```python
from build123d import *

# Parameters (mm, degrees)
SKETCH1_R           = 12
BOSS_EXTRUDE1_DEPTH = 10
SKETCH2_R           = 12
BOSS_EXTRUDE2_DEPTH = 10
SKETCH3_R           = 12
BOSS_EXTRUDE3_DEPTH = 10
CUT_EXTRUDE1_DEPTH  = 6


with BuildPart() as part:
    # Sketch1 → Boss-Extrude1 (new body)
    with BuildSketch(Plane(origin=(0, 0, 0), x_dir=(1, 0, 0), z_dir=(0, 1, 0))):
        with Locations(Location((0, 0, 0), (0, 0, 270))):
            Circle(SKETCH1_R)
    extrude(amount=BOSS_EXTRUDE1_DEPTH)

    # Sketch2 → Boss-Extrude2 (add)
    with BuildSketch(Plane(origin=(0, 10, 0), x_dir=(1, 0, 0), z_dir=(0, 1, 0))):
        with Locations(Location((6, 0, 0), (0, 0, 104.477512186))):
            Circle(SKETCH2_R)
    extrude(amount=BOSS_EXTRUDE2_DEPTH)

    # Sketch3 → Boss-Extrude3 (add)
    with BuildSketch(Plane(origin=(0, 20, 0), x_dir=(1, 0, 0), z_dir=(0, 1, 0))):
        with Locations(Location((-6, 0, 0), (0, 0, 60))):
            Circle(SKETCH3_R)
    extrude(amount=BOSS_EXTRUDE3_DEPTH)

    # Sketch4 → Cut-Extrude1 (cut)
    with BuildSketch(Plane.XZ):
        with BuildLine():
            Line((-2.180114967, -2.060849032), (-2.180114967, 2.060849032))
            ThreePointArc((-2.180114967, 2.060849032), (3, 0), (-2.180114967, -2.060849032))
        make_face()
    extrude(amount=-CUT_EXTRUDE1_DEPTH, mode=Mode.SUBTRACT)


solid = part.part
```
The model under review builds one solid part; all positions refer to its coordinate system, in mm. A direction names the side the tool comes from. Give positions to 0.01 mm unless a question says otherwise; leave off trailing zeros. Write each loop counter-clockwise with the first axis right and the second up, starting at its lowest first coordinate (ties: lowest second). Pieces come first, ordered by that corner, then holes. Notation, with made-up numbers: (47, 84) - (72, 84) arc R7 ccw to (72, 90) - close; hole circle Ø6 at (-23, -27.5). An arc over 180 degrees is marked (long way). Answer in a Markdown table with one row per item. Add a question column.
1. We need section A-A on z = 0. Write out the cut boundary in (x, y), then the cut area to 3 significant figures.
2. We need section D-D on z = -8.5. Write out the cut boundary in (x, y).
3. Wall thickness on line 1 along Y through (x, z) = (-3.5, -7.75); line 2 along X through (y, z) = (3.7, 0); line 3 along Y through (x, z) = (4.5, 6): over which ranges is each line inside the solid? List them lowest first. Write a range as [from, to].
4. Tool access review of faces 1 (the cylindrical face through (3.604, 4.93, 11.446)), 2 (the flat face through (13, 10, 0)), 3 (the cylindrical face through (15.451, 14.93, 7.395)), 4 (the flat face through (-2.5, 0, -0.2)), 5 (the flat face through (-8, 10, 0)): name each direction out of +Z, -Z, +X, -X, +Y, -Y from which nothing blocks a thin tool from reaching the whole face with its end or side.
5. We need section C-C on y = 6.5. Write out the cut boundary in (x, z).
6. Draft analysis for pull direction Z (two halves, no side actions). For faces 6 (the cylindrical face through (3, 3, 0)), 7 (the cylindrical face through (2.844, 24.93, 8.11)), 8 (the flat face through (0, 6, 0)), 9 (the flat face through (-6, 30, 0)), state which applies: +Z half, -Z half, draft (parallel to the pull), parting line (faces both ways), or undercut.
7. Insertion check: P1, Ø4, axis at x = 5, y = 6.5, coming from the +Z side; P2, Ø1.6, axis at x = 0, z = 0, coming from the -Y side; P3, Ø5, axis at x = 3, y = 6.5, coming from the -Z side. Each pin has a flat end and moves straight along its axis. Give the tip position at first contact, or say it passes through.
8. We need section B-B on x = 7. Write out the cut boundary in (y, z).
Ans:
| question | item | result |
|---|---|---|
| 1 | outline | (-18, 20) - (-6, 20) - (-6, 10) - (-12, 10) - (-12, 0) - (-2.18, 0) - (-2.18, 6) - (3, 6) - (3, 0) - (12, 0) - (12, 10) - (18, 10) - (18, 20) - (6, 20) - (6, 30) - (-18, 30) - close |
| 1 | area | 689 mm^2 |
| 2 | outline | (-14.47, 20) - (-2.47, 20) - (-2.47, 10) - (-8.47, 10) - (-8.47, 0) - (8.47, 0) - (8.47, 10) - (14.47, 10) - (14.47, 20) - (2.47, 20) - (2.47, 30) - (-14.47, 30) - close |
| 3 | line 1 | y = [0, 10], [20, 30] |
| 3 | line 2 | x = [-12, -2.18], [3, 12] |
| 3 | line 3 | y = [0, 20] |
| 4 | face 1 | -Y |
| 4 | face 2 | +X, -Y |
| 4 | face 3 | none |
| 4 | face 4 | +Z, -Z, +X, -X, -Y |
| 4 | face 5 | -X |
| 5 | outline | circle Ø24 at (0, 0) |
| 6 | face 6 | undercut |
| 6 | face 7 | parting line |
| 6 | face 8 | undercut |
| 6 | face 9 | draft |
| 7 | P1 | stops at z = 11.62 |
| 7 | P2 | stops at y = 6 |
| 7 | P3 | stops at z = -11.99 |
| 8 | outline | (0, -9.75) - (10, -9.75) - (10, -11.96) - (20, -11.96) - (20, 11.96) - (10, 11.96) - (10, 9.75) - (0, 9.75) - close |
